Design review of the part built by this model. Coordinates are the model's own, in mm. Face numbers are marked on the shaded views. A direction names the side the tool comes from. Coordinates: 2 decimals unless noted, no trailing zeros. Write each loop counter-clockwise with the first axis right and the second up, starting at its lowest first coordinate (ties: lowest second). Pieces come first, ordered by that corner, then holes.
Q1. Add section D-D, the plane z = 505. Give the boundary of the cut face in (x, y).
Q2. Add section C-C, the plane z = 649. Give the boundary of the cut face in (x, y), plus the area to 3 significant figures.
Q3. Add section A-A, the plane y = 855.5. Give the boundary of the cut face in (x, z).
Q4. The part is to be moulded in two halves that separate along X. For the marked faces 3, 4 and 5, say which applies: +X half, -X half, draft (parallel to the pull), parting line (faces both ways), or undercut.
Q5. To check wall thickness, follow probe 1 along X at (y, z) = (211, 505); probe 2 along Z at (x, y) = (-505, 532.5); probe 3 along Z at (x, y) = (-637.5, 296.5). State the ranges of each line that lie inside material, in increasing order.
Q6. Add section B-B, the plane x = -505. Give the boundary of the cut face in (y, z), plus the area to 3 significant figures.
Q7. Machinability: for the marked faces 1 and 2, which of the approach directions +Z, -Z, +X, -X, +Y, -Y give a long, thin tool a straight path to every point of the face, cutting with its end or side? Answer none if there is none.
Q8. Clearance check with a flat-ended pin moving along its axis: pin 1 Ø1.5 at (x, z) = (-600, 714.5) entering from +Y. State where the tip first meets the part, or that it passes through.
Autodesk Inventor part; units mm, degrees
ref_plane "YZ Plane" through (0, 0, 0) normal (1, 0, 0) x (0, 1, 0)
ref_plane "XZ Plane" through (0, 0, 0) normal (0, 1, 0) x (-1, 0, 0)
ref_plane "XY Plane" through (0, 0, 0) normal (0, 0, 1) x (1, 0, 0)
sketch "スケッチ1" plane through (0, 0, 0) normal (0, 1, 0) x (-1, 0, 0)
  line L0 (0, 0) -> (1010, 0)
  line L1 (1010, 0) -> (1010, 1010)
  line L2 (1010, 1010) -> (0, 1010)
  line L3 (0, 1010) -> (0, 0)
  dimension "d0" = 1010
  dimension "d1" = 1010
extrude "押し出し1" add sketch "スケッチ1" along normal blind 10
sketch "スケッチ2" plane through (0, 10, 0) normal (0, 1, 0) x (1, 0, 0)
  line L0 (-1005, -1005) -> (-5, -1005)
  line L1 (-5, -1005) -> (-5, -5)
  line L2 (-5, -5) -> (-1005, -5)
  line L3 (-1005, -5) -> (-1005, -1005)
  line L4 (-1010, 0) -> (-1010, -1010)
  line L5 (-1010, -1010) -> (0, -1010)
  line L6 (0, 0) -> (-1010, 0)
  line L7 (-1010, 0) -> (-1010, -1010)
  line L8 (-1010, -1010) -> (0, -1010)
  line L9 (0, -1010) -> (0, 0)
  dimension "d4" = 1000
  dimension "d5" = 1000
  dimension "d6" = 5
  dimension "d7" = 5
extrude "押し出し2" add sketch "スケッチ2" along normal blind 1000
sketch "スケッチ3" plane through (0, 10, 0) normal (0, 1, 0) x (1, 0, 0)
  circle A0 centre (-505, -505) radius 50
  line L0 (-1005, -1005) -> (-1005, -5)
  line L1 (-5, -1005) -> (-1005, -1005)
  circle A1 centre (-505, -505) radius 47.5
  point P0 (0, 0)
  dimension "d10" = 100
  dimension "d11" = 500
  dimension "d12" = 500
  dimension "d13" = 95
extrude "押し出し3" add sketch "スケッチ3" along normal blind 1000
properties part number "sebis-1"
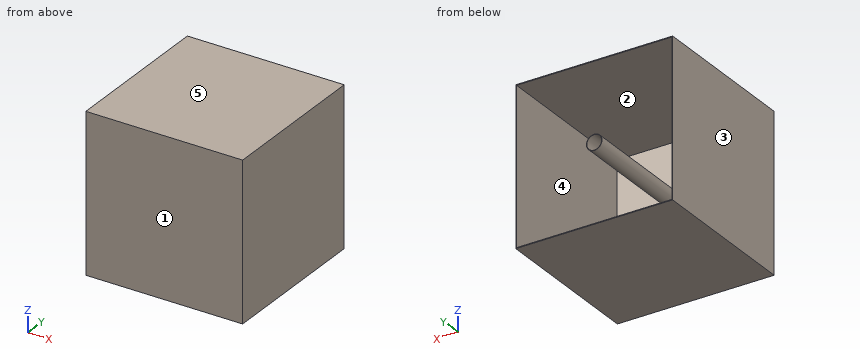
Here are the results:
1. outline: (-1010, 0) - (0, 0) - (0, 1010) - (-5, 1010) - (-5, 10) - (-455, 10) - (-455, 1010) - (-457.5, 1010) - (-457.5, 10) - (-552.5, 10) - (-552.5, 1010) - (-555, 1010) - (-555, 10) - (-1005, 10) - (-1005, 1010) - (-1010, 1010) - close
2. outline: (-1010, 0) - (0, 0) - (0, 1010) - (-5, 1010) - (-5, 10) - (-1005, 10) - (-1005, 1010) - (-1010, 1010) - close
2. area: 20,100 mm2
3. outline: (-1010, 0) - (0, 0) - (0, 1010) - (-1010, 1010) - close; circle Ø100 at (-505, 505); hole (-1005, 5) - (-5, 5) - (-5, 1005) - (-1005, 1005) - close; hole circle Ø95 at (-505, 505)
4. face 3: -X half
4. face 4: undercut
4. face 5: draft
5. probe 1: x = -1010 to -1005, -555 to -552.5, -457.5 to -455, -5 to 0
5. probe 2: z = 0 to 5, 455 to 457.5, 552.5 to 555, 1005 to 1010
5. probe 3: z = 0 to 5, 1005 to 1010
6. outline: (0, 0) - (1010, 0) - (1010, 5) - (10, 5) - (10, 455) - (1010, 455) - (1010, 457.5) - (10, 457.5) - (10, 552.5) - (1010, 552.5) - (1010, 555) - (10, 555) - (10, 1005) - (1010, 1005) - (1010, 1010) - (0, 1010) - close
6. area: 25,100 mm2
7. face 1: +Z, -Z, +X, -X, -Y
7. face 2: +Y
8. pin 1: stops at y = 10
